Source: CAD feature listing. Evaluate the final solid. Frame: model axes, mm. A direction names the side the tool comes from. Give positions to 0.01 mm unless a question says otherwise; leave off trailing zeros. Write each loop counter-clockwise with the first axis right and the second up, starting at its lowest first coordinate (ties: lowest second). Pieces come first, ordered by that corner, then holes. Notation, with made-up numbers: (11.5, 65) -> (46.5, 65) arc R26 ccw to (46.5, 82) -> close; hole circle Ø4 at (36.5, -31.5). An arc over 180 degrees is marked (long way). Write item = value, one per line.
from build123d import *

# Parameters (mm, degrees)
SKETCH002_R     = 12.5
SKETCH002_R_2   = 5
PAD003_DEPTH    = 8.8
PAD004_DEPTH    = 1
FILLET001_R     = 0.5
SKETCH008_W     = 7.8
SKETCH008_H     = 1
POCKET001_DEPTH = 9.8


with BuildPart() as part:
    # Sketch002 → Pad003 (new body)
    with BuildSketch(Plane.XY.offset(21.2)):
        Circle(SKETCH002_R)
        Circle(SKETCH002_R_2, mode=Mode.SUBTRACT)
    extrude(amount=PAD003_DEPTH)

    # Sketch005 → Pad004 (new body)
    with BuildSketch(Plane(origin=(0, 0, 21.2), x_dir=(1, 0, 0), z_dir=(0, 0, -1))):
        with BuildLine():
            ThreePointArc((12.5, 0), (0, 12.5), (-12.5, 0))
            Line((-12.5, 0), (-5, 0))
            ThreePointArc((5, 0), (0, 5), (-5, 0))
            Line((5, 0), (12.5, 0))
        make_face()
    extrude(amount=PAD004_DEPTH)

    # Fillet001
    fillet001_edges = [part.edges().sort_by_distance(p)[0] for p in [
        (-12.5, 0, 30),
    ]]
    fillet(fillet001_edges, radius=FILLET001_R)

    # Sketch008 → Pocket001 (cut)
    with BuildSketch(Plane.XY.offset(30)):
        with Locations((8.7, -0.5)):
            Rectangle(SKETCH008_W, SKETCH008_H)
    extrude(amount=-POCKET001_DEPTH, mode=Mode.SUBTRACT)


solid = part.part
1) Contact query for flat-ended pins moving along their axis: pin 1 (1.5 mm diameter, centred on y = -1.5, z = 24.5, fed in from +X); pin 2 (5 mm diameter, centred on y = -5.5, z = 23.5, fed in from +X); pin 3 (3 mm diameter, centred on x = 8, z = 27.5, fed in from +Y). Output: stop coordinate, or through.
Computed:
pin_1 = 12.46
pin_2 = 12.13
pin_3 = 10.68
2) Material intervals for L1, parallel to Y at x = 0, z = 24.75; L2, parallel to Z at x = 4.75, y = 4.5; L3, parallel to X at y = 2.25, z = 24, sorted ascending.
Computed:
L1 = -12.5 to -5, 5 to 12.5
L2 = 21.2 to 30
L3 = -12.3 to -4.47, 4.47 to 12.3
3) Cut plane A-A (x = 0). Return the cut outline in (y, z).
Computed:
outline = (-12.5, 20.2) -> (-5, 20.2) -> (-5, 30) -> (-12, 30) arc R0.5 ccw to (-12.5, 29.5) -> close; (5, 21.2) -> (12.5, 21.2) -> (12.5, 29.5) arc R0.5 ccw to (12, 30) -> (5, 30) -> close
4) Cut plane B-B (z = 22.25). Return the cut outline in (x, y).
Computed:
outline = (4.9, -1) arc R5 cw (long way) to (5, 0) -> (12.5, 0) arc R12.5 ccw (long way) to (12.46, -1) -> close
5) Access query for faces 1 (the flat face through (0, -6, 20.2)), 2 (the flat face through (-9, 0, 21)), 3 (the flat face through (9, 0, 26)). Directions: +Z, -Z, +X, -X, +Y, -Y. A direction counts if a zero-diameter tool reaches every point of the face in a straight line with its end or side. Return the directions, or none.
Computed:
face_1 = -Z, +X, -X, +Y, -Y
face_2 = -Z, +X, -X, +Y
face_3 = +Z, -Z, +X
6) Draft query along Y for faces 4 (the cylindrical face through (-2.348, -12.278, 24.915)), 5 (the cylindrical face through (-4, -3, 25)), 6 (the flat face through (5.2, 0.2, 30)). Return one class per face: pulls with the +Y half, pulls with the -Y half, needs draft (parallel to the pull), parting line crosses it, or undercut.
Computed:
face_4 = parting line crosses it
face_5 = undercut
face_6 = needs draft
